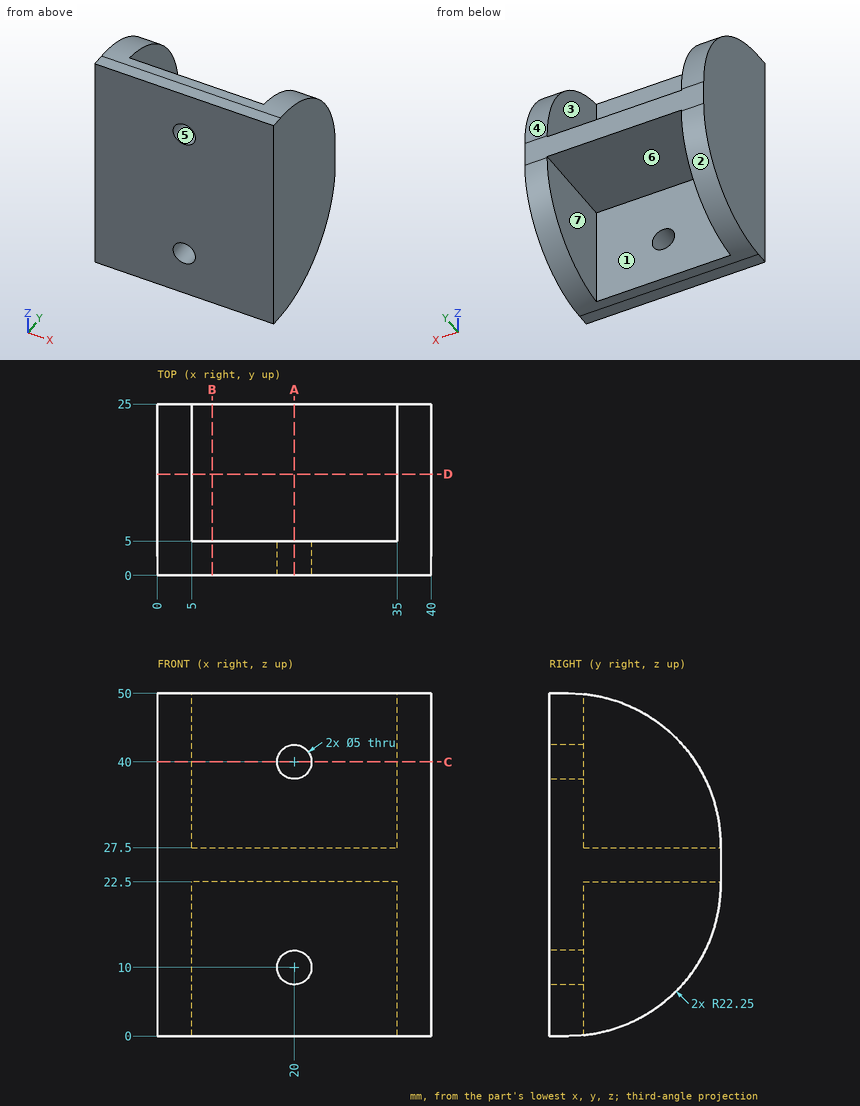
Check sheet for the drawn part. Datum: minimum x, y, z corner. Units: mm. A direction names the side the tool comes from. Give positions to 0.01 mm unless a question says otherwise; leave off trailing zeros. Order: outer loops, then holes, each group sorted by start corner. A loop starts at its lowest first (then second) coordinate and runs counter-clockwise, first axis right, second up. Notation, with made-up numbers: (-37.5, 17.5) - (9.5, 17.5) arc R30 cw to (9.5, 44.5) - close; hole circle Ø10 at (-11.5, 77.5). An arc over 180 degrees is marked (long way). Answer as a JSON object with one key per item and string values.
(1) Cross-section at D-D (y = 14.75). Record the cut outline in (x, z), then the cut area to 3 significant figures.
Report:
{"outline": "(0, 3.51) - (5, 3.51) - (5, 22.5) - (35, 22.5) - (35, 3.51) - (40, 3.51) - (40, 46.49) - (35, 46.49) - (35, 27.5) - (5, 27.5) - (5, 46.49) - (0, 46.49) - close", "area": "580 mm^2"}
(2) Cross-section at A-A (x = 20). Record the cut outline in (y, z).
Report:
{"outline": "(0, 0) - (2.75, 0) arc R22.25 ccw to (5, 0.11) - (5, 7.5) - (0, 7.5) - close; (0, 12.5) - (5, 12.5) - (5, 22.5) - (25, 22.5) - (25, 27.5) - (5, 27.5) - (5, 37.5) - (0, 37.5) - close; (0, 42.5) - (5, 42.5) - (5, 49.89) arc R22.25 ccw to (2.75, 50) - (0, 50) - close"}
(3) Depth check by flat-ended pin: pin 1 Ø2 at (x, z) = (7, 42.5) entering from -Y; pin 2 Ø3 at (x, z) = (20, 40) entering from -Y; pin 3 Ø6 at (x, y) = (13.5, 12) entering from +Z; pin 4 Ø2 at (x, y) = (7, 5) entering from +Z. Enter the tip coordinate at first touch or a pass-through.
Report:
{"pin 1": "y = 0", "pin 2": "through", "pin 3": "z = 27.5", "pin 4": "z = 49.96"}
(4) Cross-section at B-B (x = 8). Record the cut outline in (y, z), then the cut area to 3 significant figures.
Report:
{"outline": "(0, 0) - (2.75, 0) arc R22.25 ccw to (5, 0.11) - (5, 22.5) - (25, 22.5) - (25, 27.5) - (5, 27.5) - (5, 49.89) arc R22.25 ccw to (2.75, 50) - (0, 50) - close", "area": "350 mm^2"}
(5) Tool access check on the marked faces 1, 2 and 3. Record the directions out of +Z, -Z, +X, -X, +Y, -Y that give a thin tool (end or side, any length) a straight path to the whole face; none if there is none.
Report:
{"face 1": "-Z, +Y", "face 2": "-Z, +X, -X, +Y", "face 3": "+Z, +Y"}
(6) Draft check along Z on the marked faces 4, 5, 6 and 7. Enter one of: released by +Z, released by -Z, zero draft, split by the parting line, or undercut.
Report:
{"face 4": "released by +Z", "face 5": "undercut", "face 6": "released by -Z", "face 7": "zero draft"}
(7) Cross-section at C-C (z = 40). Record the cut outline in (x, y).
Report:
{"outline": "(0, 0) - (17.5, 0) - (17.5, 5) - (5, 5) - (5, 21.32) - (0, 21.32) - close; (22.5, 0) - (40, 0) - (40, 21.32) - (35, 21.32) - (35, 5) - (22.5, 5) - close"}
(8) Material ranges on line 1 (Z direction, x = 20, y = 2.1); line 2 (X direction, y = 22, z = 33.5); line 3 (Y direction, x = 25.5, z = 13.5), recorded low to high.
Report:
{"line 1": "0 to 7.5, 12.5 to 37.5, 42.5 to 50", "line 2": "0 to 5, 35 to 40", "line 3": "0 to 5"}
